Build history of the part. All positions in model axes, mm. A direction names the side the tool comes from. Round coordinates to 2 decimals unless told otherwise and drop trailing zeros. Write each loop counter-clockwise with the first axis right and the second up, starting at its lowest first coordinate (ties: lowest second). Pieces come first, ordered by that corner, then holes.
1) Saw through at D-D (y = -14.5). Write the cut outline in (x, z).
2) Saw through at B-B (x = 0). Write the cut outline in (y, z) (3 decimals), plus the area to 3 significant figures.
3) Which spindle directions (+Z, -Z, +X, -X, +Y, -Y) get a long thin tool onto all of the face, cutting with end or side? Do faces 1 (the flat face through (0, -14.986, -15)), 2 (the flat face through (12.21, -0.63, 10.1)), 3 (the cylindrical face through (-13.335, -5.009, -0.045)). Say none if no direction does.
4) Flat gauge pins, fed straight in: pin 1 (10 mm diameter, centred on x = 8.5, z = -1.5, fed in from +Y); pin 2 (0.5 mm diameter, centred on y = -15.5, z = 14.5, fed in from +X); pin 3 (1.5 mm diameter, centred on x = 15.5, z = -2.5, fed in from +Y); pin 4 (2.5 mm diameter, centred on y = -7, z = -15, fed in from +X). Where does each tip first touch, or does it go through?
5) Wall check: probe 1 along Y at (x, z) = (6, -6.5); probe 2 along Z at (x, y) = (-8, -1.5); probe 3 along X at (y, z) = (-10, 15.5). Give the ranges that are in metal, low to high.
6) Saw through at C-C (z = 0). Write the cut outline in (x, y) (3 decimals).
7) Pull direction Z, two halves, no side cores. Call faces 4 (the flat face through (-2.4, -15.5, -15)), 5 (the flat face through (13, -1.27, 9)), 6 (the flat face through (-12.305, -15.501, 8.911)), 7 (the flat face through (-12.269, -15.501, -8.874)): +Z half, -Z half, draft (parallel to the pull), parting line (faces both ways), or undercut.
Autodesk Inventor part; units mm, degrees
ref_plane "to_dummy_XY" through (0, 0, 0) normal (0, -1, 0) x (1, 0, 0)
ref_plane "to_dummy_YZ" through (0, 0, 0) normal (1, 0, 0) x (0, 0, 1)
ref_plane "to_dummy_ZX" through (0, 0, 0) normal (0, 0, 1) x (0, -1, 0)
sketch "Sketch_1" plane through (0, 0, 0) normal (1, 0, 0) x (0, 1, 0)
  line L0 (-16.002, 0) -> (0, 0)
  line L1 (0, 0) -> (0, -16.3703)
  arc A0 (-0.635, -17.0053) -> (0, -16.3703) centre (-0.635, -16.3703) ccw
  line L2 (-0.635, -17.0053) -> (-16.002, -17.0053)
  line L3 (-16.002, -17.0053) -> (-16.002, 0)
  line L4 (-16.002, 0) -> (0, 0)
revolve "Revolution1" add sketch "Sketch_1" angle 360 about axis through (0, -16.002, 0) along (0, -1, 0)
sketch "Sketch_2" plane through (0, 0, 0) normal (0, 1, 0) x (-1, 0, 0)
  circle A0 centre (0, 0) radius 21.59
  line L0 (17.78, -3.81) -> (13.4434, -3.81)
  arc A1 (12.9501, -3.1808) -> (13.4434, -3.81) centre (13.4434, -3.302) ccw
  arc A2 (12.9501, -3.1808) -> (12.9501, 3.1808) centre (0, 0) ccw
  arc A3 (13.4434, 3.81) -> (12.9501, 3.1808) centre (13.4434, 3.302) ccw
  line L1 (13.4434, 3.81) -> (17.78, 3.81)
  arc A4 (17.78, 3.81) -> (15.2664, 9.8783) centre (0, 0) ccw
  line L2 (15.2664, 9.8783) -> (12.2, 6.8119)
  arc A5 (11.4063, 6.9079) -> (12.2, 6.8119) centre (11.8408, 7.1711) ccw
  arc A6 (11.4063, 6.9079) -> (6.9079, 11.4063) centre (0, 0) ccw
  arc A7 (6.8119, 12.2) -> (6.9079, 11.4063) centre (7.1711, 11.8408) ccw
  line L3 (6.8119, 12.2) -> (9.8783, 15.2664)
  arc A8 (9.8783, 15.2664) -> (3.81, 17.78) centre (0, 0) ccw
  line L4 (3.81, 17.78) -> (3.81, 13.4434)
  arc A9 (3.1808, 12.9501) -> (3.81, 13.4434) centre (3.302, 13.4434) ccw
  arc A10 (3.1808, 12.9501) -> (-3.1808, 12.9501) centre (0, 0) ccw
  arc A11 (-3.81, 13.4434) -> (-3.1808, 12.9501) centre (-3.302, 13.4434) ccw
  line L5 (-3.81, 13.4434) -> (-3.81, 17.78)
  arc A12 (-3.81, 17.78) -> (-3.81, -17.78) centre (0, 0) ccw
  line L6 (-3.81, -17.78) -> (-3.81, -13.4434)
  arc A13 (-3.1808, -12.9501) -> (-3.81, -13.4434) centre (-3.302, -13.4434) ccw
  arc A14 (-3.1808, -12.9501) -> (3.1808, -12.9501) centre (0, 0) ccw
  arc A15 (3.81, -13.4434) -> (3.1808, -12.9501) centre (3.302, -13.4434) ccw
  line L7 (3.81, -13.4434) -> (3.81, -17.78)
  arc A16 (3.81, -17.78) -> (9.8783, -15.2664) centre (0, 0) ccw
  line L8 (9.8783, -15.2664) -> (6.8119, -12.2)
  arc A17 (6.9079, -11.4063) -> (6.8119, -12.2) centre (7.1711, -11.8408) ccw
  arc A18 (6.9079, -11.4063) -> (11.4063, -6.9079) centre (0, 0) ccw
  arc A19 (12.2, -6.8119) -> (11.4063, -6.9079) centre (11.8408, -7.1711) ccw
  line L9 (12.2, -6.8119) -> (15.2664, -9.8783)
  arc A20 (15.2664, -9.8783) -> (17.78, -3.81) centre (0, 0) ccw
extrude "Extrusion1" cut sketch "Sketch_2" against normal blind 10.16
sketch "Sketch_3" plane through (0, 0, 0) normal (0, 1, 0) x (-1, 0, 0)
  circle A0 centre (0, 0) radius 20.4599
  arc A1 (-17.2893, -4.3382) -> (-13.8361, 11.2385) centre (0, 0) ccw
  line L0 (-13.8361, 11.2385) -> (-11.2363, 9.4181)
  arc A2 (-12.6468, 7.305) -> (-11.2363, 9.4181) centre (-11.9823, 8.3888) ccw
  line L1 (-12.6468, 7.305) -> (-15.293, 9.1579)
  arc A3 (-15.293, 9.1579) -> (-17.7304, -1.8368) centre (0, 0) ccw
  line L2 (-17.7304, -1.8368) -> (-14.6049, -1.2856)
  arc A4 (-14.1081, -3.7772) -> (-14.6049, -1.2856) centre (-14.4046, -2.541) ccw
  line L3 (-14.1081, -3.7772) -> (-17.2893, -4.3382)
extrude "Extrusion2" cut sketch "Sketch_3" against normal blind 1.27
sketch "Sketch_4" plane through (0, -16.002, 0) normal (0, 1, 0) x (1, 0, 0)
  circle A0 centre (0, 0) radius 21.59
  line L0 (-17.78, 2.4003) -> (-13.1172, 2.4003)
  arc A1 (-13.1172, 2.4003) -> (-13.1172, -2.4003) centre (0, 0) ccw
  line L1 (-13.1172, -2.4003) -> (-17.78, -2.4003)
  arc A2 (-17.78, -2.4003) -> (-14.2696, -10.8751) centre (0, 0) ccw
  line L2 (-14.2696, -10.8751) -> (-10.9725, -7.578)
  arc A3 (-10.9725, -7.578) -> (-7.578, -10.9725) centre (0, 0) ccw
  line L3 (-7.578, -10.9725) -> (-10.8751, -14.2696)
  arc A4 (-10.8751, -14.2696) -> (-2.4003, -17.78) centre (0, 0) ccw
  line L4 (-2.4003, -17.78) -> (-2.4003, -13.1172)
  arc A5 (-2.4003, -13.1172) -> (2.4003, -13.1172) centre (0, 0) ccw
  line L5 (2.4003, -13.1172) -> (2.4003, -17.78)
  arc A6 (2.4003, -17.78) -> (2.4003, 17.78) centre (0, 0) ccw
  line L6 (2.4003, 17.78) -> (2.4003, 13.1172)
  arc A7 (2.4003, 13.1172) -> (-2.4003, 13.1172) centre (0, 0) ccw
  line L7 (-2.4003, 13.1172) -> (-2.4003, 17.78)
  arc A8 (-2.4003, 17.78) -> (-10.8751, 14.2696) centre (0, 0) ccw
  line L8 (-10.8751, 14.2696) -> (-7.578, 10.9725)
  arc A9 (-7.578, 10.9725) -> (-10.9725, 7.578) centre (0, 0) ccw
  line L9 (-10.9725, 7.578) -> (-14.2696, 10.8751)
  arc A10 (-14.2696, 10.8751) -> (-17.78, 2.4003) centre (0, 0) ccw
extrude "Extrusion3" cut sketch "Sketch_4" along normal blind 1.016
sketch "Sketch_8" plane through (0, 0, 0) normal (0, 1, 0) x (-1, 0, 0)
  arc A0 (3.6802, 0.9861) -> (0.9861, 3.6802) centre (0, 0) ccw
  line L0 (0.9861, 3.6802) -> (-3.6802, -0.9861)
  arc A1 (-3.6802, -0.9861) -> (-0.9861, -3.6802) centre (0, 0) ccw
  line L1 (-0.9861, -3.6802) -> (3.6802, 0.9861)
extrude "Extrusion4" add sketch "Sketch_8" against normal blind 17.78
ref_plane "to_dummy_XY" through (0, 0, 0) normal (0, -1, 0) x (1, 0, 0)
ref_plane "to_dummy_YZ" through (0, 0, 0) normal (1, 0, 0) x (0, 0, 1)
ref_plane "to_dummy_ZX" through (0, 0, 0) normal (0, 0, 1) x (0, -1, 0)
ref_plane "to_shaft_XY" through (0, 0, 0) normal (0, -1, 0) x (1, 0, 0)
ref_plane "to_shaft_YZ" through (0, 0, 0) normal (1, 0, 0) x (0, 0, 1)
ref_plane "to_shaft_ZX" through (0, 0, 0) normal (0, 0, 1) x (0, -1, 0)
ref_plane "to_trmnls_XY" through (0, -14.986, 0) normal (0, 1, 0) x (1, 0, 0)
ref_plane "to_trmnls_YZ" through (0, -14.986, 0) normal (1, 0, 0) x (0, 0, -1)
ref_plane "to_trmnls_ZX" through (0, -14.986, 0) normal (0, 0, -1) x (0, 1, 0)
properties part number "HS13Z-body"
Evaluation:
1. outline: circle Ø34.01 at (0, 0)
2. outline: (-17.78, -2.694) - (-16.002, -2.694) - (-16.002, -13.335) - (-14.986, -13.335) - (-14.986, -17.005) - (-10.16, -17.005) - (-10.16, -13.335) - (0, -13.335) - (0, 13.335) - (-10.16, 13.335) - (-10.16, 17.005) - (-14.986, 17.005) - (-14.986, 13.335) - (-16.002, 13.335) - (-16.002, 2.694) - (-17.78, 2.694) - close
2. area: 472 mm2
3. face 1: -Z, -Y
3. face 2: +X, +Y
3. face 3: -X, +Y
4. pin 1: stops at y = 0
4. pin 2: stops at x = 9.28
4. pin 3: stops at y = -1.27
4. pin 4: stops at x = 10.01
5. probe 1: y = -16 to 0
5. probe 2: z = -15.01 to -13.39, -10.67 to 10.67, 13.39 to 15.01
5. probe 3: x = -7 to -3.81, 3.81 to 7
6. outline: (-17.005, -14.986) - (-13.335, -14.986) - (-13.335, -16.002) - (-2.694, -16.002) - (-2.694, -17.78) - (2.694, -17.78) - (2.694, -16.002) - (17.005, -16.002) - (17.005, -0.635) arc R0.635 ccw to (16.37, 0) - (-13.335, 0) - (-13.335, -10.16) - (-17.005, -10.16) - close
7. face 4: draft
7. face 5: undercut
7. face 6: +Z half
7. face 7: -Z half
